Check sheet for the drawn part. Datum: minimum x, y, z corner. Units: mm. A direction names the side the tool comes from. Give positions to 0.01 mm unless a question says otherwise; leave off trailing zeros. Write each loop counter-clockwise with the first axis right and the second up, starting at its lowest first coordinate (ties: lowest second). Pieces come first, ordered by that corner, then holes. Notation, with made-up numbers: M 14.5,11 L 23.5,11 A37 cw 23.5,49 Z; hole C -17,-12.75 d6. An arc over 180 degrees is marked long. Write item = value, one per line.
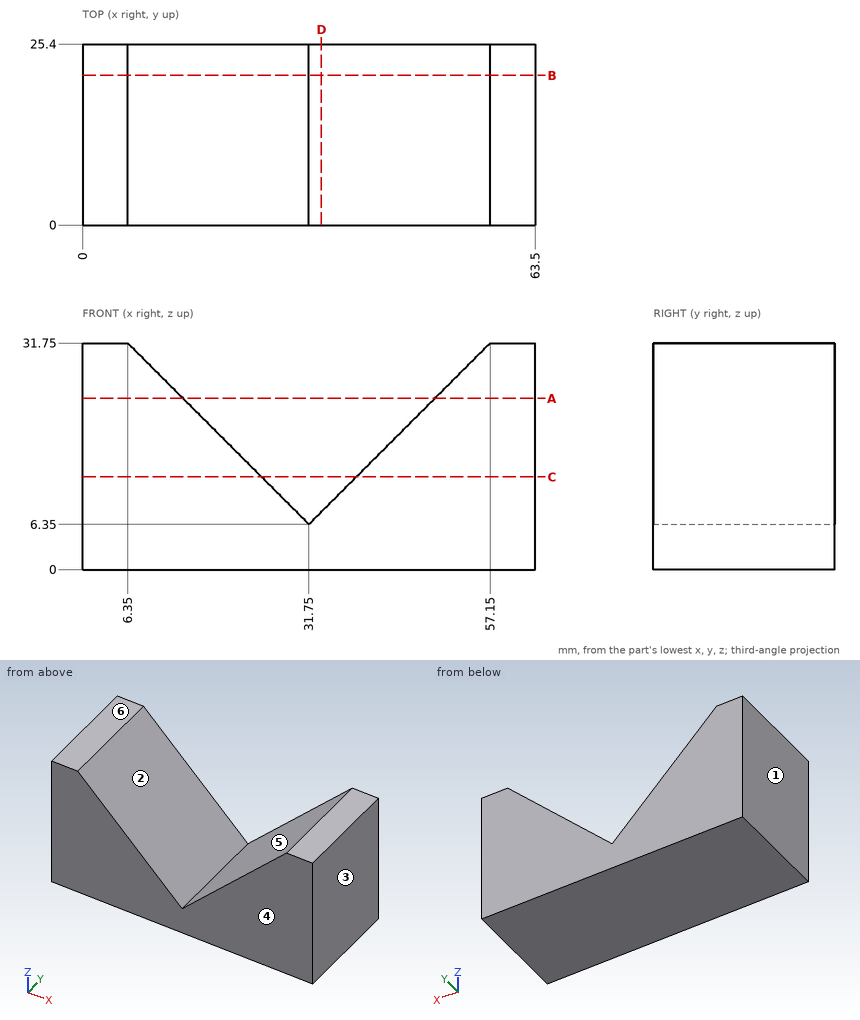
1) Cross-section at A-A on z = 24. Record the boundary of the cut face in (x, y), plus the area to 3 significant figures.
From the geometry:
outline = M 0,0 L 14.1,0 L 14.1,25.4 L 0,25.4 Z; M 49.4,0 L 63.5,0 L 63.5,25.4 L 49.4,25.4 Z
area = 716 mm^2
2) Draft check along X on the marked faces 1, 2, 3 and 4. Enter one of: +X half, -X half, draft (parallel to the pull), parting line (faces both ways), or undercut.
From the geometry:
face_1 = -X half
face_2 = undercut
face_3 = +X half
face_4 = draft
3) Cross-section at B-B on y = 21. Record the boundary of the cut face in (x, z).
From the geometry:
outline = M 0,0 L 63.5,0 L 63.5,31.75 L 57.15,31.75 L 31.75,6.35 L 6.35,31.75 L 0,31.75 Z
4) Material ranges on probe 1 along X at (y, z) = (22, 6.5); probe 2 along X at (y, z) = (14.75, 17); probe 3 along Z at (x, y) = (55, 11.75), recorded low to high. Write a range as from..to.
From the geometry:
probe_1 = 0..31.6, 31.9..63.5
probe_2 = 0..21.1, 42.4..63.5
probe_3 = 0..29.6
5) Cross-section at D-D on x = 33.5. Record the boundary of the cut face in (y, z).
From the geometry:
outline = M 0,0 L 25.4,0 L 25.4,8.1 L 0,8.1 Z
6) Tool access check on the marked faces 5 and 6. Record the directions out of +Z, -Z, +X, -X, +Y, -Y that give a thin tool (end or side, any length) a straight path to the whole face; none if there is none.
From the geometry:
face_5 = +Z, +Y, -Y
face_6 = +Z, +X, -X, +Y, -Y
7) Depth check by flat-ended pin: P1, Ø1, axis at x = 40, y = 3.5, coming from the +Z side; P2, Ø10, axis at y = 18.5, z = 28.5, coming from the -X side; P3, Ø1.5, axis at x = 31.5, y = 10.5, coming from the +Z side; P4, Ø2, axis at x = 27, y = 3.5, coming from the +Z side. Enter the tip coordinate at first touch or a pass-through.
From the geometry:
P1 = 15.1
P2 = 0
P3 = 7.35
P4 = 12.1
8) Cross-section at C-C on z = 13. Record the boundary of the cut face in (x, y).
From the geometry:
outline = M 0,0 L 25.1,0 L 25.1,25.4 L 0,25.4 Z; M 38.4,0 L 63.5,0 L 63.5,25.4 L 38.4,25.4 Z
